Here's how the part is built. I have some questions about the finished solid (model axes, mm). A direction names the side the tool comes from. Coordinates: 2 decimals unless noted, no trailing zeros. Write each loop counter-clockwise with the first axis right and the second up, starting at its lowest first coordinate (ties: lowest second). Pieces come first, ordered by that corner, then holes. Notation, with made-up numbers: (27, 15) -> (50, 15) arc R26 cw to (50, 35) -> close; hole circle Ø4 at (39.25, -16.75). An arc over 180 degrees is marked (long way). Put each result on its own line as item: value.
```python
from build123d import *

# Parameters (mm, degrees)
SKETCH1_W               = 70
SKETCH1_H               = 40
BOSS_EXTRUDE1_DEPTH     = 30
SKETCH3_W               = 20
SKETCH3_H               = 30
CUT_EXTRUDE1_DEPTH      = 1
CUT_EXTRUDE1_DEPTH_BACK = 31
SKETCH4_W               = 35
SKETCH4_H               = 20
CUT_EXTRUDE2_DEPTH      = 41
SKETCH5_R               = 5
CUT_EXTRUDE3_DEPTH      = 30
SKETCH6_W               = 20
SKETCH6_H               = 10
CUT_EXTRUDE4_DEPTH      = 11
SKETCH7_R               = 5
CUT_EXTRUDE5_DEPTH      = 30


with BuildPart() as part:
    # Sketch1 → Boss-Extrude1 (new body)
    with BuildSketch(Plane(origin=(0, 0, 0), x_dir=(1, 0, 0), z_dir=(0, 1, 0))):
        with Locations((35, 20)):
            Rectangle(SKETCH1_W, SKETCH1_H)
    extrude(amount=BOSS_EXTRUDE1_DEPTH)

    # Sketch3 → Cut-Extrude1 (cut, two sides)
    with BuildSketch(Plane(origin=(0, 30, 0), x_dir=(1, 0, 0), z_dir=(0, 1, 0))) as cut_extrude1_sk:
        with Locations((60, 15)):
            Rectangle(SKETCH3_W, SKETCH3_H)
    extrude(amount=CUT_EXTRUDE1_DEPTH, mode=Mode.SUBTRACT)
    extrude(cut_extrude1_sk.sketch, amount=-CUT_EXTRUDE1_DEPTH_BACK, mode=Mode.SUBTRACT)

    # Sketch4 → Cut-Extrude2 (cut, through all)
    with BuildSketch(Plane.XY):
        with Locations((17.5, 20)):
            Rectangle(SKETCH4_W, SKETCH4_H)
    extrude(amount=-CUT_EXTRUDE2_DEPTH, mode=Mode.SUBTRACT)

    # Sketch5 → Cut-Extrude3 (cut)
    with BuildSketch(Plane(origin=(50, 0, 0), x_dir=(0, 0, -1), z_dir=(1, 0, 0))):
        with Locations((15, 20)):
            Circle(SKETCH5_R)
    extrude(amount=-CUT_EXTRUDE3_DEPTH, mode=Mode.SUBTRACT)

    # Sketch6 → Cut-Extrude4 (cut, through all)
    with BuildSketch(Plane(origin=(0, 10, 0), x_dir=(1, 0, 0), z_dir=(0, 1, 0))):
        with Locations((10, 5)):
            Rectangle(SKETCH6_W, SKETCH6_H)
    extrude(amount=-CUT_EXTRUDE4_DEPTH, mode=Mode.SUBTRACT)

    # Sketch7 → Cut-Extrude5 (cut)
    with BuildSketch(Plane(origin=(0, 10, 0), x_dir=(1, 0, 0), z_dir=(0, 1, 0))):
        with Locations((15, 25)):
            Circle(SKETCH7_R)
    extrude(amount=-CUT_EXTRUDE5_DEPTH, mode=Mode.SUBTRACT)


solid = part.part
```
Item 1: If we mould it in two halves opening along X, with no side actions, what happens to faces 1 (the cylindrical face through (17.307, 5.07, -20.564)), 2 (the flat face through (50, 12, -15)), 3 (the flat face through (27, 0, -25))? For each: released by +X, released by -X, zero draft, split by the parting line, or undercut.
Output:
face 1: undercut
face 2: released by +X
face 3: zero draft
Item 2: Imagine slicing it at C-C on x = 15. Write out the boundary of the cut face in (y, z), then the cut area to 3 significant figures.
Output:
outline: (0, -40) -> (10, -40) -> (10, -30) -> (0, -30) -> close; (0, -20) -> (10, -20) -> (10, -10) -> (0, -10) -> close
area: 200 mm²
Item 3: For P1, Ø10, axis at x = 62, y = 13, coming from the +Z side; P2, Ø8, axis at y = 26.5, z = -12, coming from the +X side; P3, Ø5, axis at x = 10, y = 5, coming from the +Z side, each with a flat end and sliding along its axis, tell me the tip position at first contact or that it passes through.
Output:
P1: stops at z = -30
P2: stops at x = 50
P3: stops at z = -10
Item 4: Please list where these lines run through material, in increasing order: line 1 along Z through (x, y) = (15, 7.25); line 2 along X through (y, z) = (7.5, -25); line 3 along X through (y, z) = (22.75, -23). Write a range as from..to.
Output:
line 1: z = -40..-30, -20..-10
line 2: x = 0..10, 20..50
line 3: x = 35..50
Item 5: Imagine slicing it at D-D on y = 20. Write out the boundary of the cut face in (x, z), then the cut area to 3 significant figures.
Output:
outline: (35, -40) -> (70, -40) -> (70, -30) -> (50, -30) -> (50, -20) -> (35, -20) -> close; (35, -10) -> (50, -10) -> (50, 0) -> (35, 0) -> close
area: 650 mm²
Item 6: Imagine slicing it at B-B on y = 5.75. Write out the boundary of the cut face in (x, z).
Output:
outline: (0, -40) -> (70, -40) -> (70, -30) -> (50, -30) -> (50, 0) -> (20, 0) -> (20, -10) -> (0, -10) -> close; hole circle Ø10 at (15, -25)
Item 7: Imagine slicing it at A-A on z = -25. Write out the boundary of the cut face in (x, y).
Output:
outline: (0, 0) -> (10, 0) -> (10, 10) -> (0, 10) -> close; (20, 0) -> (50, 0) -> (50, 30) -> (35, 30) -> (35, 10) -> (20, 10) -> close
Item 8: Which directions (+Z, -Z, +X, -X, +Y, -Y) give clear straight access to the entire face, cutting with the end or side of a thin tool? Please do faces 4 (the cylindrical face through (42.605, 15.564, -17.307)), 5 (the flat face through (60, 15, -30)), 6 (the flat face through (0, 5, -25)), 7 (the flat face through (17, 10, -20)), 8 (the flat face through (10, 5, -10)).
Output:
face 4: +X, -X
face 5: +Z, +X, +Y, -Y
face 6: +Z, -Z, -X, +Y, -Y
face 7: +Z, -Z, -X, +Y
face 8: +Z, -X, +Y, -Y
